from build123d import *

# Parameters (mm, degrees)
MODEL_R                 = 1.5
SALIENTE_EXTRUIR1_DEPTH = 3


with BuildPart() as part:
    # Model → Saliente-Extruir1 (new body)
    with BuildSketch(Plane.XY):
        with BuildLine():
            Line((139.599121875, 257.495671711), (133.599121875, 257.495671711))
            ThreePointArc((133.599121875, 257.495671711), (131.87704643, 257.153129607), (130.41714136, 256.177652227))
            Line((130.41714136, 256.177652227), (124.053180329, 249.813691196))
            ThreePointArc((124.053180329, 249.813691196), (124.053180329, 243.449730165), (130.41714136, 243.449730165))
            Line((130.41714136, 243.449730165), (134.145063421, 247.177652226))
            ThreePointArc((134.145063421, 247.177652226), (135.604968491, 248.153129607), (137.327043937, 248.495671711))
            Line((137.327043937, 248.495671711), (138.099121875, 248.495671711))
            Line((138.099121875, 248.495671711), (139.599121875, 248.495671711))
            ThreePointArc((139.599121875, 248.495671711), (144.099121875, 252.995671711), (139.599121875, 257.495671711))
        make_face()
        with Locations((133.599121875, 252.995671711)):
            Circle(MODEL_R, mode=Mode.SUBTRACT)
        with Locations((127.235160845, 246.631710681)):
            Circle(MODEL_R, mode=Mode.SUBTRACT)
    extrude(amount=SALIENTE_EXTRUIR1_DEPTH)


solid = part.part
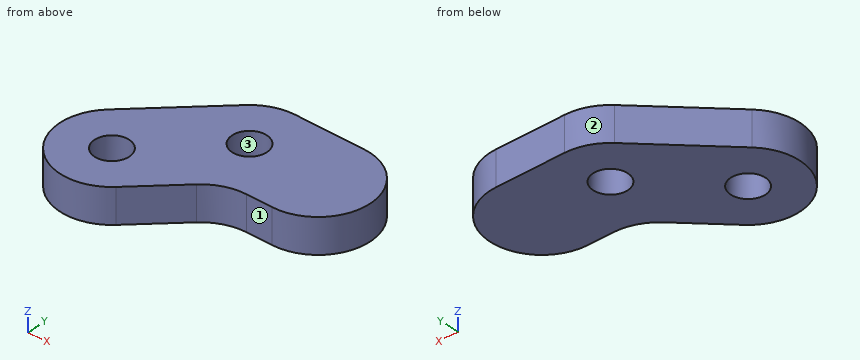
Could you check a few things on this model? Use its own coordinates, in mm. Face numbers are marked on the shaded views. Coordinates: 2 decimals unless noted, no trailing zeros. Order: outer loops, then holes, each group sorted by start corner. A loop starts at its lowest first (then second) coordinate and runs counter-clockwise, first axis right, second up. Notation, with made-up numbers: (55.25, 53.25) - (73.25, 53.25) arc R32 ccw to (73.25, 81.25) - close; hole circle Ø11 at (-9, 83). An arc over 180 degrees is marked (long way). Answer in a Markdown table with one row per item. Add a question column.
(1) I need wall thicknesses on L1, parallel to Y at x = 133, z = 1.1; L2, parallel to X at y = 253, z = 1.85; L3, parallel to Y at x = 132, z = 2.25. Which ranges of each line are inside material? Lowest first, please.
(2) Will this pin go through, and if not, where does the flat tip stop? pin 1 (1.5 mm diameter, centred on y = 246.5, z = 0.5, fed in from +X).
(3) If we mould it in two halves opening along X, with no side actions, what happens to the marked faces 1, 2 and 3? For each: released by +X, released by -X, zero draft, split by the parting line, or undercut.
(4) If we section it at A-A, the plane y = 247.75: Please give me the cut outline in (x, z).
(5) If we section it at D-D, the plane x = 138.5: Please give me the cut outline in (y, z).
(6) If we section it at B-B, the plane x = 126.5: Please give me the cut outline in (y, z).
(7) If we section it at C-C, the plane z = 0.9: Please give me the cut outline in (x, y), then the cut area to 3 significant figures.
Results are:
| question | item | result |
|---|---|---|
| 1 | L1 | y = 246.03 to 251.62, 254.37 to 257.46 |
| 1 | L2 | x = 127.24 to 132.1, 135.1 to 144.1 |
| 1 | L3 | y = 245.03 to 257.2 |
| 2 | pin 1 | stops at x = 134.22 |
| 3 | face 1 | zero draft |
| 3 | face 2 | released by -X |
| 3 | face 3 | undercut |
| 4 | outline | (122.88, 0) - (126.24, 0) - (126.24, 3) - (122.88, 3) - close; (128.23, 0) - (134.85, 0) - (134.85, 3) - (128.23, 3) - close |
| 5 | outline | (248.5, 0) - (257.5, 0) - (257.5, 3) - (248.5, 3) - close |
| 6 | outline | (242.19, 0) - (245.32, 0) - (245.32, 3) - (242.19, 3) - close; (247.94, 0) - (252.26, 0) - (252.26, 3) - (247.94, 3) - close |
| 7 | outline | (124.05, 249.81) arc R4.5 ccw to (130.42, 243.45) - (134.15, 247.18) arc R4.5 cw to (137.33, 248.5) - (139.6, 248.5) arc R4.5 ccw to (139.6, 257.5) - (133.6, 257.5) arc R4.5 ccw to (130.42, 256.18) - close; hole circle Ø3 at (127.24, 246.63); hole circle Ø3 at (133.6, 253) |
| 7 | area | 184 mm2 |
